Autodesk Fusion 360 part; units mm, degrees
sketch "Sketch1" plane through (0, 0, 0) normal (0, 1, 0) x (1, 0, 0)
  line L0 (-48.8546, -55.3051) -> (-1.7146, -55.3051)
  line L1 (-1.7146, -55.3051) -> (-1.7146, 10.0349)
  line L2 (-1.7146, 10.0349) -> (-48.8546, 10.0349)
  line L3 (-48.8546, 10.0349) -> (-48.8546, -55.3051)
  line L4 (-58.8546, -65.3051) -> (8.2854, -65.3051)
  line L5 (8.2854, -65.3051) -> (8.2854, 20.0349)
  line L6 (8.2854, 20.0349) -> (-58.8546, 20.0349)
  line L7 (-58.8546, 20.0349) -> (-58.8546, -65.3051)
  circle A0 centre (-53.8546, -60.3051) radius 1.45
  circle A1 centre (-53.8546, 15.0349) radius 1.45
  circle A2 centre (3.2854, 15.0349) radius 1.45
  circle A3 centre (3.2854, -60.3051) radius 1.45
  dimension "d1" = 47.14
  dimension "d2" = 65.34
  dimension "d3" = 10
  dimension "d4" = 10
  dimension "d5" = 10
  dimension "d6" = 10
  dimension "d7" = 2.9
  dimension "d8" = 5
  dimension "d9" = 5
  dimension "d10" = 2.9
  dimension "d11" = 5
  dimension "d12" = 5
  dimension "d13" = 2.9
  dimension "d14" = 5
  dimension "d15" = 5
  dimension "d16" = 2.9
  dimension "d17" = 5
  dimension "d18" = 5
extrude "Extrude1" add sketch "Sketch1" along normal blind 10 contours L0 L1 L2 L3 | L4 L5 L6 L7
sketch "Sketch2" plane through (0, 0, 0) normal (0, 1, 0) x (1, 0, 0)
  line L0 (-48.8399, -56.2293) -> (-1.6999, -56.2293)
  line L1 (-1.6999, -56.2293) -> (-1.6999, 9.1107)
  line L2 (-1.6999, 9.1107) -> (-48.8399, 9.1107)
  line L3 (-48.8399, 9.1107) -> (-48.8399, -56.2293)
  dimension "d21" = 47.14
  dimension "d22" = 65.34
extrude "Extrude2" cut sketch "Sketch2" along normal blind 7
extrude "Extrude3" add 1 faces at (-33.1363, 0, -13.4796) along direction (0, -1, 0) blind 3
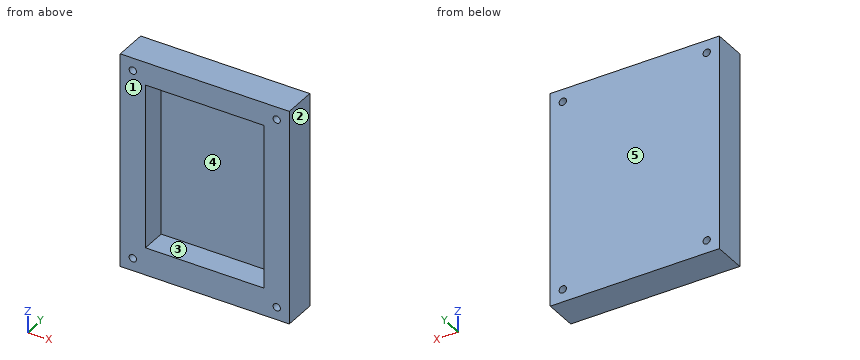
Geometry check sheet. Reference: the model listing, model coordinates, mm. Face numbers are marked on the shaded views. A direction names the side the tool comes from. Coordinates: 2 decimals unless noted, no trailing zeros. Order: outer loops, then holes, each group sorted by start corner. A loop starts at its lowest first (then second) coordinate and runs counter-clockwise, first axis right, second up. Notation, with made-up numbers: (69, 78.25) -> (119, 78.25) arc R4 cw to (119, 83.25) -> close; hole circle Ø4 at (22, 75.5). An arc over 180 degrees is marked (long way). Use a Markdown table: item, result. Add a question column.
1. Mould release check, pull along X, two halves, no side actions. Record for the marked faces 1, 2 and 3: pulls with the +X half, pulls with the -X half, needs draft (parallel to the pull), parting line crosses it, or undercut.
2. Cross-section at C-C (z = 26). Enter the section's corners in (x, y).
3. Cross-section at A-A (x = -14). Enter the section's corners in (y, z), and give its area (3 significant figures).
4. Cross-section at B-B (y = 5.5). Enter the section's corners in (x, z).
5. Go/stop test with flat-tipped pins: pin 1 Ø1.7 at (x, z) = (3.29, -15.03) entering from -Y; pin 2 Ø14 at (x, z) = (-31.5, 18.5) entering from -Y. Record where each tip stops, or that it passes through.
6. Material ranges on L1, parallel to X at y = 5, z = 49; L2, parallel to Z at x = -25.5, y = 5.75; L3, parallel to Z at x = -54.5, y = 8.75, recorded low to high.
7. Set-up check for the marked faces 4 and 5: record each of +Z, -Z, +X, -X, +Y, -Y from which the full face is reachable in a straight line by a thin tool's end or side.
Filled sheet:
| question | item | result |
|---|---|---|
| 1 | face 1 | needs draft |
| 1 | face 2 | pulls with the +X half |
| 1 | face 3 | undercut |
| 2 | outline | (-58.85, -3) -> (-48.84, -3) -> (-48.84, 7) -> (-1.7, 7) -> (-1.7, -3) -> (8.29, -3) -> (8.29, 10) -> (-58.85, 10) -> close |
| 3 | outline | (-3, -20.03) -> (10, -20.03) -> (10, 65.31) -> (-3, 65.31) -> (-3, 56.23) -> (7, 56.23) -> (7, -9.11) -> (-3, -9.11) -> close |
| 3 | area | 456 mm2 |
| 4 | outline | (-58.85, -20.03) -> (8.29, -20.03) -> (8.29, 65.31) -> (-58.85, 65.31) -> close; hole circle Ø2.9 at (-53.85, -15.03); hole circle Ø2.9 at (-53.85, 60.31); hole (-48.84, -9.11) -> (-1.7, -9.11) -> (-1.7, 56.23) -> (-48.84, 56.23) -> close; hole circle Ø2.9 at (3.29, -15.03); hole circle Ø2.9 at (3.29, 60.31) |
| 5 | pin 1 | through |
| 5 | pin 2 | y = 7 |
| 6 | L1 | -58.85 to -48.84, -1.7 to 8.29 |
| 6 | L2 | -20.03 to -9.11, 56.23 to 65.31 |
| 6 | L3 | -20.03 to -16.33, -13.74 to 59.01, 61.6 to 65.31 |
| 7 | face 4 | -Y |
| 7 | face 5 | +Z, -Z, +X, -X, +Y |
